Could you check a few things on this model? Use its own coordinates, in mm. Face numbers are marked on the shaded views. A direction names the side the tool comes from. Coordinates: 2 decimals unless noted, no trailing zeros. Write each loop counter-clockwise with the first axis right and the second up, starting at its lowest first coordinate (ties: lowest second). Pieces come first, ordered by that corner, then holes.
Item 1: I want a section at B-B on z = 8.75. Please give me the cut outline in (x, y) (1 decimal), then the cut area to 3 significant figures.
Item 2: If I drill on probe 1 along Z at (x, y) = (5, -44); probe 2 along Y at (x, z) = (5, 17.5); probe 3 along Y at (x, z) = (-26.5, 18.5), over which ranges is the centre line in solid material (lowest first)?
Item 3: Which directions (+Z, -Z, +X, -X, +Y, -Y) give clear straight access to the entire face, cutting with the end or side of a thin tool? Please do the marked faces 1 and 2.
Item 4: For P1, Ø1.5, axis at y = 10, z = 9, coming from the +X side; P2, Ø2, axis at y = -19.5, z = 12, coming from the +X side; P3, Ø6, axis at x = -15.5, z = 13, coming from the -Y side; P4, Ø2.5, axis at x = 5, z = 5, coming from the +Y side, each with a flat end and sliding along its axis, tell me the tip position at first contact or that it passes through.
Item 5: I want a section at C-C on y = 11. Please give me the cut outline in (x, z), then the cut area to 3 significant figures.
Item 6: I want a section at D-D on x = -6. Please give me the cut outline in (y, z).
Item 7: I want a section at A-A on x = 5. Please give me the cut outline in (y, z) (1 decimal), then the cut area to 4 significant figures.
Autodesk Inventor part; units mm, degrees
ref_plane "YZ Plane" through (0, 0, 0) normal (1, 0, 0) x (0, 1, 0)
ref_plane "XZ Plane" through (0, 0, 0) normal (0, 1, 0) x (-1, 0, 0)
ref_plane "XY Plane" through (0, 0, 0) normal (0, 0, 1) x (1, 0, 0)
sketch "Sketch1" plane through (0, 0, 0) normal (0, 0, 1) x (1, 0, 0)
  arc A0 (-30.4516, 17.5812) -> (0, -35.1625) centre (0, 0) ccw
  line L0 (0, 0) -> (30.1625, 0)
  line L1 (0, 0) -> (17.5813, 30.4516)
  line L2 (0, 0) -> (-30.4516, 17.5812)
  line L3 (0, -30.1625) -> (0, -35.1625)
  arc A1 (-26.1215, 15.0812) -> (0, -30.1625) centre (0, 0) ccw
  arc A2 (30.1625, 0) -> (15.0813, 26.1215) centre (0, 0) ccw
  line L4 (0, -30.1625) -> (30.1625, -30.1625)
  line L5 (30.1625, -30.1625) -> (30.1625, -42.6625)
  line L6 (30.1625, -42.6625) -> (0, -42.6625)
  line L7 (0, -42.6625) -> (0, -30.1625)
  line L8 (0, -42.6625) -> (10, -42.6625)
  line L9 (10, -42.6625) -> (10, -47.6625)
  line L10 (10, -47.6625) -> (0, -47.6625)
  line L11 (0, -47.6625) -> (0, -42.6625)
  line L12 (0, -47.6625) -> (0, -35.1625)
  line L13 (0, -47.6625) -> (-5, -47.6625)
  line L14 (-5, -47.6625) -> (-5, -42.6625)
  line L15 (-5, -42.6625) -> (0, -42.6625)
  line L16 (0, -42.6625) -> (0, -47.6625)
  line L17 (-5, -47.6625) -> (-26.4528, -23.1657)
  line L18 (0, -42.6625) -> (0, -35.1625)
  dimension "d3" = 60
  dimension "d4" = 30.1625
  dimension "d5" = 35.1625
  dimension "d6" = 12.5
  dimension "d7" = 10
  dimension "d8" = 5
extrude "Extrusion1" add sketch "Sketch1" along normal blind 20 contours L2 A1 L3 A0 | A0 L7 L15 L14 L17 | L14 L15 L11 L13 | L6 L9 L10 L11
sketch "Sketch2" plane through (-5, -47.6625, 0) normal (0, -1, 0) x (1, 0, 0)
  line L0 (0, 0) -> (15, 0)
  line L1 (15, 0) -> (15, 20)
  line L2 (0, 20) -> (15, 20)
  line L3 (0, 0) -> (0, 20)
  line L4 (10, 20) -> (10, 0)
  circle A0 centre (10, 15) radius 1.6
  circle A1 centre (10, 5) radius 1.6
  point P0 (5, 0)
  dimension "d11" = 3.2
  dimension "d13" = 5
  dimension "d14" = 5
  dimension "d15" = 5
extrude "Extrusion2" cut sketch "Sketch2" against normal through all contours A1 L4 | L4 A1 | A0 L4 | L4 A0
sketch "Sketch3" plane through (-5, -47.6625, 0) normal (0, -1, 0) x (1, 0, 0)
  circle A0 centre (10, 5) radius 1.6
  circle A1 centre (10, 15) radius 1.6
  line L0 (6.738, 15) -> (8.369, 17.825)
  line L1 (8.369, 17.825) -> (11.631, 17.825)
  line L2 (11.631, 17.825) -> (13.262, 15)
  line L3 (13.262, 15) -> (11.631, 12.175)
  line L4 (11.631, 12.175) -> (8.369, 12.175)
  line L5 (8.369, 12.175) -> (6.738, 15)
  line L6 (6.738, 5) -> (8.369, 7.825)
  line L7 (8.369, 7.825) -> (11.631, 7.825)
  line L8 (11.631, 7.825) -> (13.262, 5)
  line L9 (13.262, 5) -> (11.631, 2.175)
  line L10 (11.631, 2.175) -> (8.369, 2.175)
  line L11 (8.369, 2.175) -> (6.738, 5)
  point P0 (5, 0)
  dimension "d18" = 5.65
extrude "Extrusion3" cut sketch "Sketch3" against normal blind 2.5
properties part number "clip"
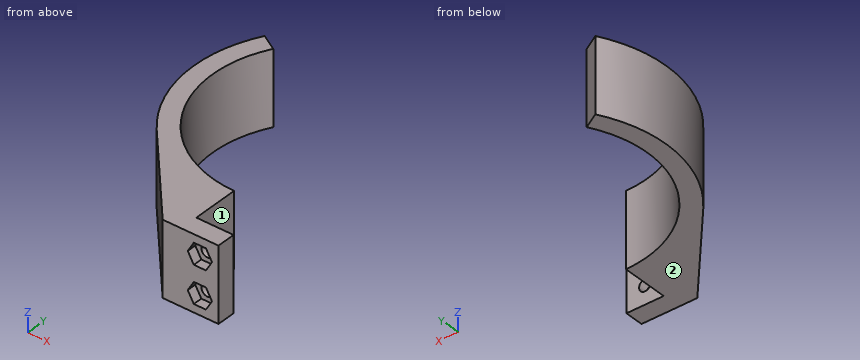
Response values:
1. outline: (-30.5, 17.6) arc R35.2 ccw to (-26.5, -23.2) - (-5, -47.7) - (10, -47.7) - (10, -42.7) - (0, -42.7) - (0, -30.2) arc R30.2 cw to (-26.1, 15.1) - close
1. area: 557 mm2
2. probe 1: z = 0 to 3.4, 6.6 to 13.4, 16.6 to 20
2. probe 2: y = -45.16 to -42.66
2. probe 3: y = -23.11 to -14.41, 14.41 to 15.3
3. face 1: +Z, -Z, +X, +Y
3. face 2: -Z, +X, -X, +Y, -Y
4. P1: stops at x = -28.18
4. P2: stops at x = -22.13
4. P3: stops at y = -39.1
4. P4: passes through
5. outline: (-33.4, 0) - (-28.09, 0) - (-28.09, 20) - (-33.4, 20) - close
5. area: 106 mm2
6. outline: (-46.52, 0) - (-29.56, 0) - (-29.56, 20) - (-46.52, 20) - close
7. outline: (-47.7, 0) - (-42.7, 0) - (-42.7, 3.4) - (-45.2, 3.4) - (-45.2, 2.2) - (-47.7, 2.2) - close; (-47.7, 7.8) - (-45.2, 7.8) - (-45.2, 6.6) - (-42.7, 6.6) - (-42.7, 13.4) - (-45.2, 13.4) - (-45.2, 12.2) - (-47.7, 12.2) - close; (-47.7, 17.8) - (-45.2, 17.8) - (-45.2, 16.6) - (-42.7, 16.6) - (-42.7, 20) - (-47.7, 20) - close
7. area: 55.75 mm2
